Model file for the job. Use its own axes, mm. Give positions to 0.01 mm unless a question says otherwise; leave off trailing zeros. Write each loop counter-clockwise with the first axis right and the second up, starting at its lowest first coordinate (ties: lowest second). Pieces come first, ordered by that corner, then holes. Notation, with made-up numbers: (80, 41) - (85, 41) arc R19 cw to (85, 69) - close; hole circle Ø8 at (53.5, 30). An arc over 180 degrees is marked (long way). Use CSV: the item, a comma, the result in double quotes.
from build123d import *

# Parameters (mm, degrees)
SKETCH1_R          = 103
BASE_DISC_DEPTH    = 1.5
SKETCH3_R          = 3
CUT_EXTRUDE1_DEPTH = 146.671719973
SKETCH4_RX         = 28
SKETCH4_RY         = 16
CUT_EXTRUDE2_DEPTH = 146.671719973
SKETCH2_R          = 7.5
CUT_EXTRUDE3_DEPTH = 146.671720116
CIRPATTERN3_COUNT  = 4
CIRPATTERN4_COUNT  = 4
SKETCH5_R          = 1.4
CUT_EXTRUDE4_DEPTH = 146.671720116


with BuildPart() as part:
    # Sketch1 → Base Disc (new body)
    with BuildSketch(Plane.XY):
        Circle(SKETCH1_R)
    extrude(amount=BASE_DISC_DEPTH)

    # Sketch3 → Cut-Extrude1 (cut, through all)
    with BuildSketch(Plane(origin=(0, 0, 0), x_dir=(-1, 0, 0), z_dir=(0, 0, -1))):
        with Locations((95, 0)):
            Circle(SKETCH3_R)
    cut_extrude1 = extrude(amount=-CUT_EXTRUDE1_DEPTH, mode=Mode.SUBTRACT)

    # Sketch4 → Cut-Extrude2 (cut, through all)
    with BuildSketch(Plane(origin=(0, 0, 0), x_dir=(-1, 0, 0), z_dir=(0, 0, -1))):
        with Locations(Location((38.890872965, 38.890872965), (0, 0, 135))):
            Ellipse(SKETCH4_RX, SKETCH4_RY)
    cut_extrude2 = extrude(amount=-CUT_EXTRUDE2_DEPTH, mode=Mode.SUBTRACT)

    # Sketch2 → Cut-Extrude3 (cut, through all)
    with BuildSketch(Plane(origin=(0, 0, 0), x_dir=(-1, 0, 0), z_dir=(0, 0, -1))):
        Circle(SKETCH2_R)
    extrude(amount=-CUT_EXTRUDE3_DEPTH, mode=Mode.SUBTRACT)

    # CirPattern3: Cut-Extrude1 ×4 about axis
    cirpattern3_axis = Axis((0, 0, 0), (0, 0, 1))
    for i in range(1, CIRPATTERN3_COUNT):
        add(cut_extrude1.rotate(cirpattern3_axis, i * 360 / CIRPATTERN3_COUNT), mode=Mode.SUBTRACT)

    # CirPattern4: Cut-Extrude2 ×4 about axis
    cirpattern4_axis = Axis((0, 0, 0), (0, 0, -1))
    for i in range(1, CIRPATTERN4_COUNT):
        add(cut_extrude2.rotate(cirpattern4_axis, i * 360 / CIRPATTERN4_COUNT), mode=Mode.SUBTRACT)

    # Sketch5 → Cut-Extrude4 (cut, through all)
    with BuildSketch(Plane.XY):
        with Locations((-7.778174593, -7.778174593)):
            Circle(SKETCH5_R)
        with Locations((-7.778174593, 7.778174593)):
            Circle(SKETCH5_R)
        with Locations((7.778174593, 7.778174593)):
            Circle(SKETCH5_R)
        with Locations((7.778174593, -7.778174593)):
            Circle(SKETCH5_R)
    extrude(amount=CUT_EXTRUDE4_DEPTH, mode=Mode.SUBTRACT)


solid = part.part
(1) Pull direction X, two halves, no side cores. Call faces 1 (the face through (-22.33, -100.55, 0.74)), 2 (the face through (0, 92, 1)), 3 (the face through (-1, -21, 1.5)): released by +X, released by -X, zero draft, split by the parting line, or undercut.
Checked values:
face 1,"split by the parting line"
face 2,"undercut"
face 3,"zero draft"
(2) Saw through at A-A, the plane y = 0. List the corners of the cut face in (x, z), then the cut area to 4 significant figures.
Checked values:
outline,"(-103, 0) - (-98, 0) - (-98, 1.5) - (-103, 1.5) - close; (-92, 0) - (-7.5, 0) - (-7.5, 1.5) - (-92, 1.5) - close; (7.5, 0) - (92, 0) - (92, 1.5) - (7.5, 1.5) - close; (98, 0) - (103, 0) - (103, 1.5) - (98, 1.5) - close"
area,"268.5 mm^2"
(3) Wall check: probe 1 along Y at (x, z) = (-20.5, 1); probe 2 along X at (y, z) = (51, 0.6); probe 3 along X at (y, z) = (-46, 0.55). Give the ranges that are in metal, low to high. Write a range as [from, to].
Checked values:
probe 1,"y = [-100.94, -59.84], [-36.61, 36.61], [59.84, 100.94]"
probe 2,"x = [-89.49, -49.39], [-16.1, 16.1], [49.39, 89.49]"
probe 3,"x = [-92.16, -53.95], [-16.61, 16.61], [53.95, 92.16]"
(4) Saw through at C-C, the plane x = 95. List the corners of the cut face in (y, z), then the cut area to 3 significant figures.
Checked values:
outline,"(-39.8, 0) - (-3, 0) - (-3, 1.5) - (-39.8, 1.5) - close; (3, 0) - (39.8, 0) - (39.8, 1.5) - (3, 1.5) - close"
area,"110 mm^2"
